Part print with two shaded views. Sizes in mm from the minimum x, y, z corner. A direction names the side the tool comes from. Coordinates: 2 decimals unless noted, no trailing zeros. Loops run counter-clockwise (first coordinate to the right, second up) from the corner with the lowest first, then second, coordinate; pieces in that order, holes last.
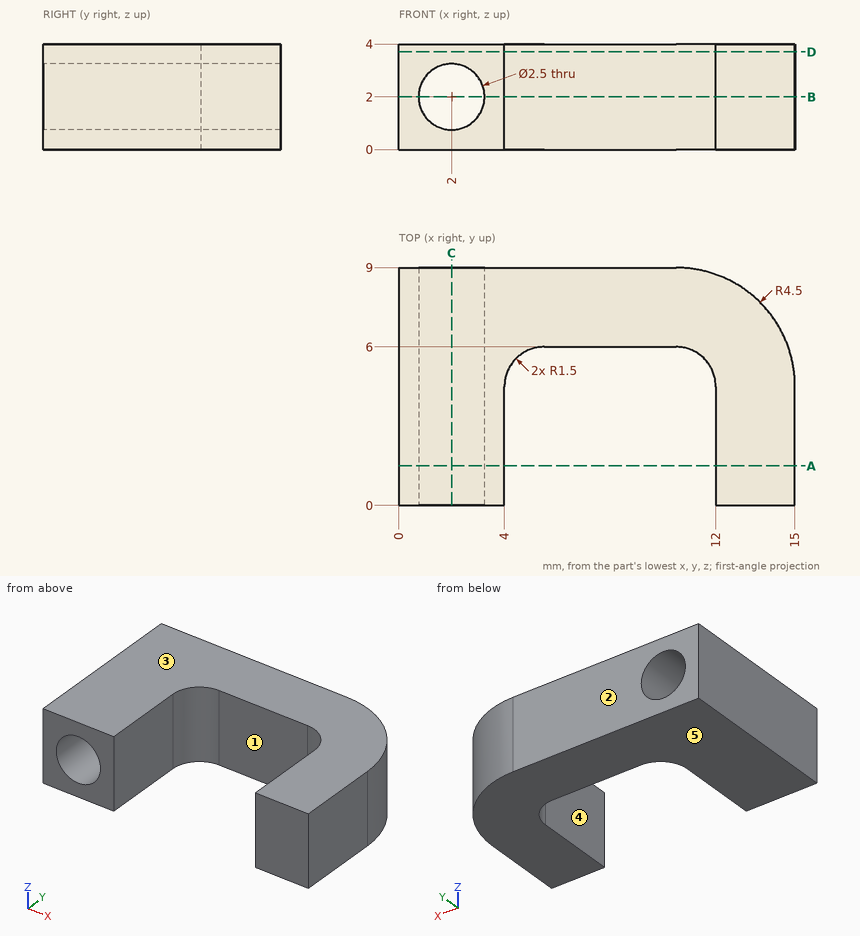
Q1. Mould opens along Y. For the marked faces 1, 2 and 3 say: +Y half, -Y half, draft (parallel to the pull), parting line (faces both ways), or undercut.
Answers:
face 1: -Y half
face 2: +Y half
face 3: draft
Q2. Slice it at B-B (z = 2). List the corners of the cut face in (x, y), and give its area (3 significant figures).
Answers:
outline: (0, 0) - (0.75, 0) - (0.75, 9) - (0, 9) - close; (3.25, 0) - (4, 0) - (4, 4.5) arc R1.5 cw to (5.5, 6) - (10.5, 6) arc R1.5 cw to (12, 4.5) - (12, 0) - (15, 0) - (15, 4.5) arc R4.5 ccw to (10.5, 9) - (3.25, 9) - close
area: 61.1 mm2
Q3. Drill centre lines: line 1 (X direction, y = 3.5, z = 2.05); line 2 (Z direction, x = 2, y = 4.25); line 3 (X direction, y = 3, z = 2.5). Where is each one in solid material? Low to high.
Answers:
line 1: x = 0 to 0.75, 3.25 to 4, 12 to 15
line 2: z = 0 to 0.75, 3.25 to 4
line 3: x = 0 to 0.85, 3.15 to 4, 12 to 15
Q4. Slice it at A-A (y = 1.5). List the corners of the cut face in (x, z).
Answers:
outline: (0, 0) - (4, 0) - (4, 4) - (0, 4) - close; (12, 0) - (15, 0) - (15, 4) - (12, 4) - close; hole circle Ø2.5 at (2, 2)
Q5. Which spindle directions (+Z, -Z, +X, -X, +Y, -Y) get a long thin tool onto all of the face, cutting with end or side? Do the marked faces 4 and 5. Say none if no direction does.
Answers:
face 4: +Z, -Z, -Y
face 5: -Z, +X, -X, +Y, -Y
Q6. Flat gauge pin, fed straight in: P1, Ø1.2, axis at x = 7, z = 2, coming from the -Y side. Where does the tip first touch, or does it go through?
Answers:
P1: stops at y = 6
Q7. Slice it at C-C (x = 2). List the corners of the cut face in (y, z).
Answers:
outline: (0, 0) - (9, 0) - (9, 0.75) - (0, 0.75) - close; (0, 3.25) - (9, 3.25) - (9, 4) - (0, 4) - close
Q8. Slice it at D-D (z = 3.7). List the corners of the cut face in (x, y), and give its area (3 significant figures).
Answers:
outline: (0, 0) - (4, 0) - (4, 4.5) arc R1.5 cw to (5.5, 6) - (10.5, 6) arc R1.5 cw to (12, 4.5) - (12, 0) - (15, 0) - (15, 4.5) arc R4.5 ccw to (10.5, 9) - (0, 9) - close
area: 83.6 mm2
